The drawing under review shows one solid part. Ordinate dimensions are in mm from its lowest x, y, z. A direction names the side the tool comes from. Give positions to 0.01 mm unless a question says otherwise; leave off trailing zeros. Loops run counter-clockwise (first coordinate to the right, second up) from the corner with the lowest first, then second, coordinate; pieces in that order, holes last.
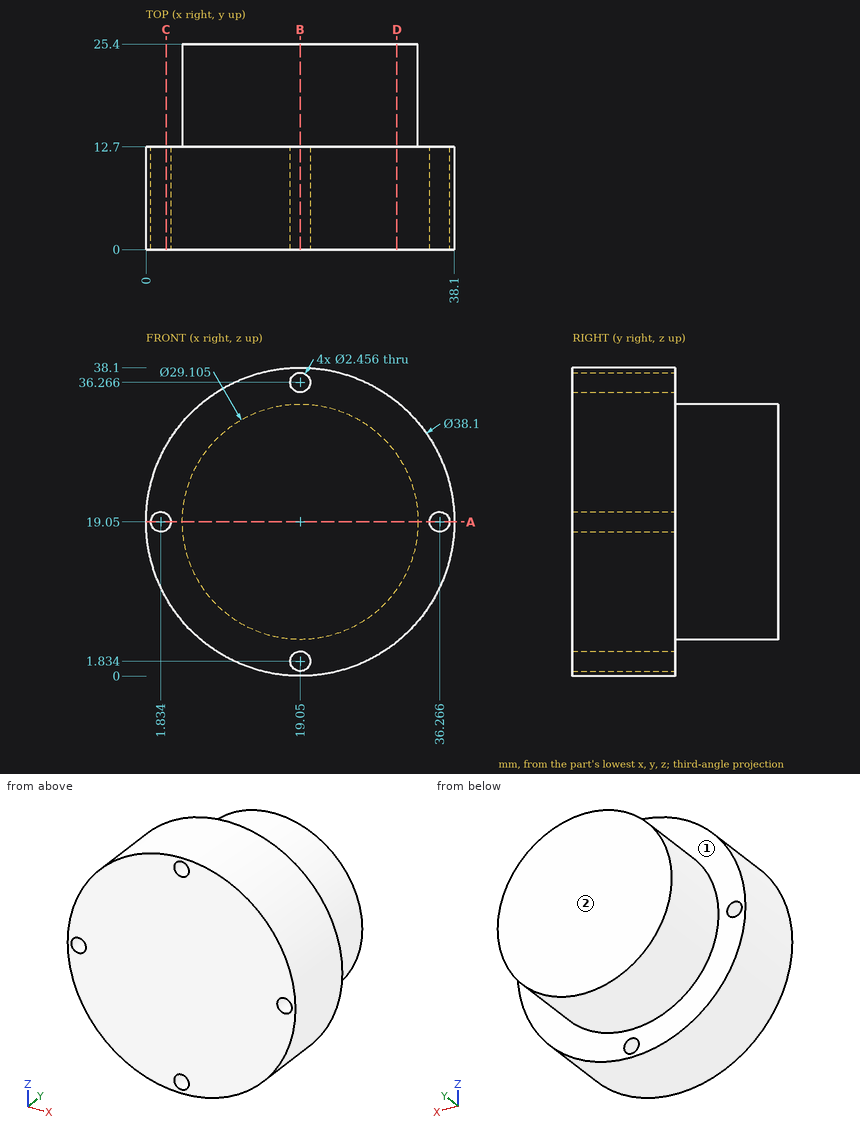
Item 1: For L1, parallel to Z at x = 19.05, y = 7.75 (1 decimal); L2, parallel to Z at x = 36.5, y = 8.75 (1 decimal); L3, parallel to Y at x = 4, z = 14, list the stretches that pass through material, from the lowest coordinate up.
Answer:
L1: z = 0 to 0.6, 3.1 to 35, 37.5 to 38.1
L2: z = 11.4 to 17.8, 20.3 to 26.7
L3: y = 0 to 12.7
Item 2: Take a section at C-C on x = 2.5. Give the boundary of the cut face in (y, z), and give its area (3 significant figures).
Answer:
outline: (0, 9.62) - (12.7, 9.62) - (12.7, 18.02) - (0, 18.02) - close; (0, 20.08) - (12.7, 20.08) - (12.7, 28.48) - (0, 28.48) - close
area: 213 mm2
Item 3: Tool access review of the marked faces 1 and 2: name each direction out of +Z, -Z, +X, -X, +Y, -Y from which nothing blocks a thin tool from reaching the whole face with its end or side.
Answer:
face 1: +Y
face 2: +Z, -Z, +X, -X, +Y
Item 4: Take a section at D-D on x = 31. Give the boundary of the cut face in (y, z) (1 decimal).
Answer:
outline: (0, 4.2) - (12.7, 4.2) - (12.7, 10.7) - (25.4, 10.7) - (25.4, 27.4) - (12.7, 27.4) - (12.7, 33.9) - (0, 33.9) - close
Item 5: Clearance check with flat-ended pins moving along their axes: pin 1 Ø12 at (x, z) = (30, 28) entering from -Y; pin 2 Ø3 at (x, z) = (36.27, 19.05) entering from +Y; pin 3 Ø3 at (y, z) = (13, 25.5) entering from -X; pin 4 Ø6 at (x, y) = (11.5, 6.5) entering from +Z. State where each tip first meets the part, or that it passes through.
Answer:
pin 1: stops at y = 0
pin 2: stops at y = 12.7
pin 3: stops at x = 0.66
pin 4: stops at z = 37.55
Item 6: Take a section at B-B on x = 19.05. Give the boundary of the cut face in (y, z) (1 decimal), and give its area (3 significant figures).
Answer:
outline: (0, 0) - (12.7, 0) - (12.7, 0.6) - (0, 0.6) - close; (0, 3.1) - (12.7, 3.1) - (12.7, 4.5) - (25.4, 4.5) - (25.4, 33.6) - (12.7, 33.6) - (12.7, 35) - (0, 35) - close; (0, 37.5) - (12.7, 37.5) - (12.7, 38.1) - (0, 38.1) - close
area: 791 mm2
Item 7: Take a section at A-A on z = 19.05. Give the boundary of the cut face in (x, y) (1 decimal).
Answer:
outline: (0, 0) - (0.6, 0) - (0.6, 12.7) - (0, 12.7) - close; (3.1, 0) - (35, 0) - (35, 12.7) - (33.6, 12.7) - (33.6, 25.4) - (4.5, 25.4) - (4.5, 12.7) - (3.1, 12.7) - close; (37.5, 0) - (38.1, 0) - (38.1, 12.7) - (37.5, 12.7) - close
